Could you check a few things on this model? Use its own coordinates, in mm. A direction names the side the tool comes from. Coordinates: 2 decimals unless noted, no trailing zeros. Loops run counter-clockwise (first coordinate to the right, second up) from the corner with the lowest first, then second, coordinate; pieces in that order, holes last. Notation, with made-up numbers: (68, -2) -> (95, -2) arc R20 ccw to (95, 36) -> close; hole circle Ø3 at (85, 42). An arc over 180 degrees is marked (long way). One line per question, with ' | ' between items.
from build123d import *

# Parameters (mm, degrees)
EXTRUDE_1_DEPTH      = 7.5
EXTRUDE_1_DEPTH_BACK = 7.5


with BuildPart() as part:
    # Sketch 1 → Revolve 1 (revolve)
    with BuildSketch(Plane(origin=(0, 0, 0), x_dir=(1, 0, 0), z_dir=(0, 1, 0)), mode=Mode.PRIVATE) as revolve_1_sk:
        Polygon((4, 0), (17.5, 0), (17.5, 0.9), (21.589095178, 0.9), (24, 0.254), (24, 1.910441889), (21.8, 2.499930112), (21.8, 19.500069888), (24, 20.089558111), (24, 21.746), (21.589095178, 21.1), (17.5, 21.1), (17.5, 22), (4, 22), align=None)
    revolve(revolve_1_sk.sketch.rotate(Axis((0, 0, 50), (0, 0, -1)), 180), axis=Axis((0, 0, 50), (0, 0, -1)))

    # Sketch 2 → Extrude 1 (add, two sides: drawn at the far end of the back side and taken through both)
    with BuildSketch(Plane.XY.offset(-11).offset(-EXTRUDE_1_DEPTH_BACK)):
        with BuildLine():
            Line((-86.797485344, 42.169146754), (-14.940905306, -17.87901979))
            ThreePointArc((-14.940905306, -17.87901979), (19.518784167, -12.724270691), (10.32945325, 20.885219548))
            Line((10.32945325, 20.885219548), (-73.609178047, 62.399754064))
            ThreePointArc((-73.609178047, 62.399754064), (-89.186627274, 58.140649425), (-86.797485344, 42.169146754))
        make_face()
        with BuildLine():
            Line((-84.610854997, 44.78577583), (-12.754274959, -15.262390713))
            ThreePointArc((-12.754274959, -15.262390713), (16.662172407, -10.862049101), (8.817717817, 17.828627331))
            Line((8.817717817, 17.828627331), (-75.120913479, 59.343161847))
            ThreePointArc((-75.120913479, 59.343161847), (-86.330015513, 56.278427835), (-84.610854997, 44.78577583))
        make_face(mode=Mode.SUBTRACT)
    extrude(amount=EXTRUDE_1_DEPTH + EXTRUDE_1_DEPTH_BACK)

    # Sketch 3 → Revolve 2 (revolve)
    with BuildSketch(Plane(origin=(0, 51.5, 0), x_dir=(1, 0, 0), z_dir=(0, 1, 0)), mode=Mode.PRIVATE) as revolve_2_sk:
        Polygon((-89.66, 2.5), (-87, 2.5), (-87, 0), (-83, 0), (-83, 22), (-87, 22), (-87, 19.5), (-89.66, 19.5), align=None)
    revolve(revolve_2_sk.sketch.rotate(Axis((-79, 51.5, -50), (0, 0, 1)), 180), axis=Axis((-79, 51.5, -50), (0, 0, 1)))


solid = part.part
1) I need wall thicknesses on line 1 along Y through (x, z) = (-79, -7.5); line 2 along Y through (x, z) = (0, -15.5); line 3 along Y through (x, z) = (-73, -15). Which ranges of each line are inside material? Lowest first, please. Write a range as from..to.
Data:
line 1: 35.65..40.1, 40.84..47.5, 55.5..63.66 | line 2: -23.3..-4, 4..21.8, 22.19..25.99 | line 3: 30.64..35.08, 42.69..62.1
2) I'm going to push flat-ended pins straight in: pin 1 Ø4 at (x, z) = (-36, -17) entering from -Y; pin 2 Ø1.5 at (y, z) = (7.5, -17) entering from +X; pin 3 Ø9 at (x, y) = (0, 0) entering from -Z; pin 4 Ø3 at (x, z) = (-37.5, -17.5) entering from -Y. Where does each tip first touch, or does it pass through?
Data:
pin 1: y = -1.95 | pin 2: x = 22.3 | pin 3: z = -22 | pin 4: y = -0.28
3) If we section it at C-C on y = 25.5: Please give me the cut outline in (x, z), and give its area (3 significant figures).
Data:
outline: (-66.85, -18.5) -> (-61.53, -18.5) -> (-61.53, -3.5) -> (-66.85, -3.5) -> close; (-6.69, -18.5) -> (1, -18.5) -> (1, -3.5) -> (-6.69, -3.5) -> close | area: 195 mm²
4) If we section it at A-A on z = -13.75: Please give me the cut outline in (x, y).
Data:
outline: (-86.8, 42.17) -> (-14.94, -17.88) arc R23.3 ccw (long way) to (10.33, 20.89) -> (-73.61, 62.4) arc R12.16 ccw to start; hole circle Ø8 at (-79, 51.5); hole (-79.94, 40.88) -> (-19.6, -9.54) arc R21.8 cw to (0.82, 21.78) -> (-69.66, 56.64) arc R10.66 cw to start; hole circle Ø8 at (0, 0)
5) On a 3-axis mill with a long thin cutter (end or side, diameter ignored), from which of +Z, -Z, +X, -X, +Y, -Y can I reach the whole of each face in a straight line? I mean faces 5 (the face through (-80.041, 59.432, -1.232)), 6 (the face through (-83, 59, -19.5)), 7 (the face through (-43, 7, -3.5)), 8 (the face through (-79.867, 47.595, -11.154)). Say none if no direction works.
Data:
face 5: +Z | face 6: -Z | face 7: none | face 8: +Z, -Z
6) If we section it at B-B on y = 51.5: Please give me the cut outline in (x, z).
Data:
outline: (-91.16, -18.5) -> (-89.66, -18.5) -> (-89.66, -19.5) -> (-87, -19.5) -> (-87, -22) -> (-83, -22) -> (-83, 0) -> (-87, 0) -> (-87, -2.5) -> (-89.66, -2.5) -> (-89.66, -3.5) -> (-91.16, -3.5) -> close; (-75, -22) -> (-71, -22) -> (-71, -19.5) -> (-68.34, -19.5) -> (-68.34, -2.5) -> (-71, -2.5) -> (-71, 0) -> (-75, 0) -> close; (-59.26, -18.5) -> (-51.57, -18.5) -> (-51.57, -3.5) -> (-59.26, -3.5) -> close
7) We'd pull the mould along X, two halves only. Please class faces 1 (the face through (3.794, -17.084, -21.556)), 2 (the face through (-50.19, 16.02, -11.1)), 3 (the face through (-51.372, 12.565, -11.105)), 4 (the face through (4, -4, 0)): pulls with the +X half, pulls with the -X half, needs draft (parallel to the pull), parting line crosses it, or undercut.
Data:
face 1: undercut | face 2: undercut | face 3: pulls with the -X half | face 4: needs draft
8) If we section it at D-D on y = 0: Give the number of separate pieces and of enclosed holes in the cut face, and give its area (3 significant figures).
Data:
separate pieces: 3 | enclosed holes: 0 | area: 885 mm²
